The listing builds one solid part. Answer for the finished solid, in the listing's coordinates (mm). Face numbers are marked on the shaded views. A direction names the side the tool comes from. Round coordinates to 2 decimals unless told otherwise and drop trailing zeros. Write each loop counter-clockwise with the first axis right and the second up, starting at its lowest first coordinate (ties: lowest second). Pieces come first, ordered by that corner, then holes. Notation, with made-up numbers: (29, 65) - (64, 65) arc R21 ccw to (64, 82) - close; hole circle Ø7 at (24.25, 51.25). An arc over 180 degrees is marked (long way). Return JSON: item names as keys, results as strings. Group by question number.
(1) Section C-C, the plane y = 50 is taken. Write down the section's boundary in (x, z) (3 decimals).
(2) Section B-B, the plane z = -3.5 is taken. Write down the section's boundary in (x, y) (3 decimals).
(3) Each of these flat-tipped pins is pushed along its axis until it touches: pin 1 (10 mm diameter, centred on x = 0.5, y = -30, fed in from +Z) (3 decimals); pin 2 (1.5 mm diameter, centred on y = 20.5, z = 36, fed in from +X); pin 3 (5 mm diameter, centred on x = 27, y = 7, fed in from +Z). Where does it stop, or does it pass through?
(4) Section A-A, the plane y = 11 is taken. Write down the section's boundary in (x, z) (3 decimals).
(5) Which of the six approach directions +Z, -Z, +X, -X, +Y, -Y give full straight-line access (tool end or side, diameter ignored) to the marked faces 1, 2, 3, 4 and 5?
(6) Find the intervals of material crossed by line 1 along Z through (x, y) = (57.5, -1.5); line 2 along Y through (x, z) = (-3.5, 32.5) (3 decimals); line 3 along X through (y, z) = (17, 18.5) (3 decimals), in increasing order. Write a range as [from, to].
```python
from build123d import *

# Parameters (mm, degrees)
F1_DEPTH = 63.5
F0_W     = 25.4
F0_H     = 19.05
F2_DEPTH = 25.4
F3_DEPTH = 15.875


with BuildPart() as f1:
    # F0 (on Front) → F1 (new body, symmetric)
    with BuildSketch(Plane.XZ):
        Polygon((41.275, -9.525), (41.275, 9.525), (22.225, 9.525), (-41.275, 9.525), (-41.275, -9.525), align=None)
    extrude(amount=F1_DEPTH, both=True)

    # F0 (on Front) → F2 (join, symmetric)
    with BuildSketch(Plane.XZ):
        with BuildLine():
            Line((22.225, 9.525), (41.275, 9.525))
            Line((41.275, 9.525), (41.275, 27.0002))
            ThreePointArc((41.275, 27.0002), (45.9246798487, 38.2255201513), (57.15, 42.8752))
            Line((57.15, 42.8752), (60.325, 42.8752))
            Line((60.325, 42.8752), (60.325, 61.9252))
            Line((60.325, 61.9252), (57.15, 61.9252))
            ThreePointArc((57.15, 61.9252), (32.4542956671, 51.6959043329), (22.225, 27.0002))
            Line((22.225, 27.0002), (22.225, 9.525))
        make_face()
        with Locations((73.025, 52.4002)):
            Rectangle(F0_W, F0_H)
    extrude(amount=F2_DEPTH, both=True)

    # F0 (on Front) → F3 (join)
    with BuildSketch(Plane.XZ):
        with BuildLine():
            Line((-41.275, 9.525), (22.225, 9.525))
            Line((22.225, 9.525), (22.225, 27.0002))
            ThreePointArc((22.225, 27.0002), (32.4542956671, 51.6959043329), (57.15, 61.9252))
            add(Edge.make_bspline(
                [(-41.275, 9.525), (-39.9924255908, 47.1598803997), (14.5989470184, 62.7080574632), (57.15, 61.9252)],
                knots=[0, 0, 0, 0, 111.5045361635, 111.5045361635, 111.5045361635, 111.5045361635], degree=3))
        make_face()
    extrude(amount=F3_DEPTH)


solid = f1.part
```
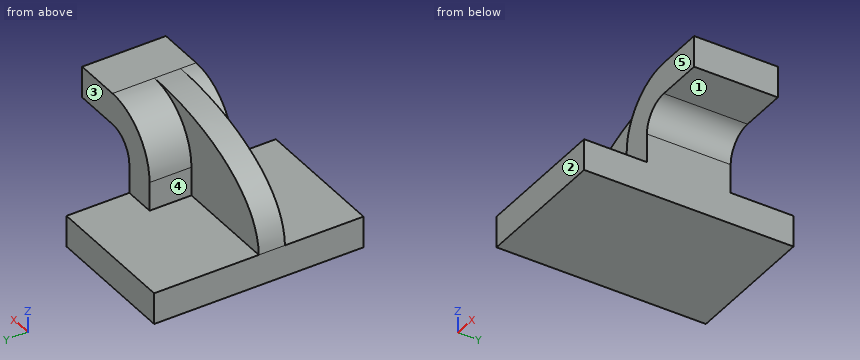
Working result:
{
 "1": {"outline": "(-41.275, -9.525) - (41.275, -9.525) - (41.275, 9.525) - (-41.275, 9.525) - close"},
 "2": {"outline": "(-41.275, -63.5) - (41.275, -63.5) - (41.275, 63.5) - (-41.275, 63.5) - close"},
 "3": {"pin 1": "stops at z = 9.525", "pin 2": "stops at x = 44.62", "pin 3": "stops at z = 48.34"},
 "4": {"outline": "(-41.275, -9.525) - (41.275, -9.525) - (41.275, 27) arc R15.875 cw to (57.15, 42.875) - (85.725, 42.875) - (85.725, 61.925) - (57.15, 61.925) arc R34.925 ccw to (22.225, 27) - (22.225, 9.525) - (-41.275, 9.525) - close"},
 "5": {"face 1": "-Z, +X, +Y, -Y", "face 2": "+Z, -Z, +X, -X, -Y", "face 3": "+Z, +X, -X, +Y", "face 4": "+Z, -X, +Y", "face 5": "+Z, +X, -X, -Y"},
 "6": {"line 1": "z = [42.88, 61.93]", "line 2": "y = [-15.875, 0]", "line 3": "x = [22.225, 41.275]"}
}
